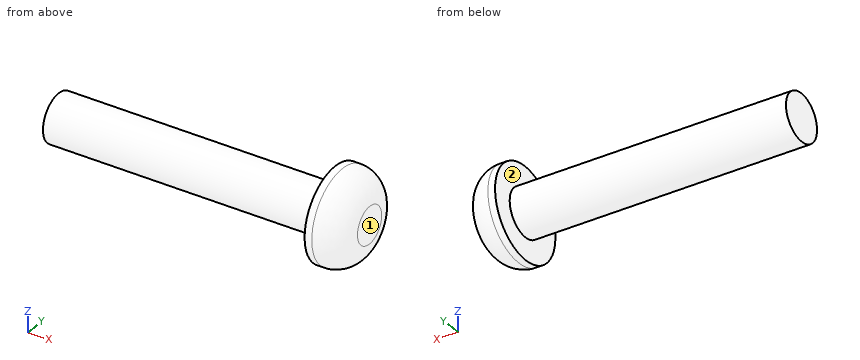
Autodesk Inventor part; units mm, degrees
ref_plane "YZ Plane" through (0, 0, 0) normal (1, 0, 0) x (0, 1, 0)
ref_plane "XZ Plane" through (0, 0, 0) normal (0, 1, 0) x (-1, 0, 0)
ref_plane "XY Plane" through (0, 0, 0) normal (0, 0, 1) x (1, 0, 0)
sketch "Sketch1" plane through (0, 0, 0) normal (1, 0, 0) x (0, 1, 0)
  circle A0 centre (0, 0) radius 1.0922
  dimension "d0" = 2.1844
extrude "Extrusion1" add sketch "Sketch1" along normal blind 12.7
sketch "Sketch2" plane through (12.7, 0, 0) normal (1, 0, 0) x (0, 0, -1)
  circle A0 centre (0, 0) radius 2.1209
  dimension "d3" = 4.2418
extrude "Extrusion2" add sketch "Sketch2" along normal blind 1.6002
fillet "Fillet1" radius 1.27 1 edges at (14.3002, 0, 2.1209)
thread "Thread1"
properties part number "2-56 screw"
Source: CAD feature listing. Evaluate the final solid. Frame: model axes, mm. Face numbers are marked on the shaded views. A direction names the side the tool comes from. Round coordinates to 2 decimals unless told otherwise and drop trailing zeros. Loops run counter-clockwise (first coordinate to the right, second up) from the corner with the lowest first, then second, coordinate; pieces in that order, holes last. Notation, with made-up numbers: M -9.75,-18 L 19.25,-18 A33 ccw 19.25,15 Z; hole C 27,-15.75 d11. An arc over 180 degrees is marked long. Return JSON: item names as keys, results as strings. Group by question number.
1. Section query A-A on x = 9.5. Output: boundary loops of the cut face in (y, z).
2. Pin query (flat end, axial travel): pin 1 (2 mm diameter, centred on x = 2.5, y = -0.5, fed in from -Z); pin 2 (1.3 mm diameter, centred on y = 0, z = 0, fed in from -X); pin 3 (1.5 mm diameter, centred on x = 5.5, z = -1, fed in from +Y). Return the tip coordinate at first contact, or that it passes through.
3. Reachability of the marked faces 1 and 2 from +Z, -Z, +X, -X, +Y, -Y: full face, straight path, thin tool, end or side. Return the list, or none.
4. Material intervals for line 1 along X through (y, z) = (-0.05, -0.9); line 2 along Y through (x, z) = (13, 0.1); line 3 along X through (y, z) = (0.75, 1.2), sorted ascending. Write a range as from..to.
Checks:
{
 "1": {"outline": "C 0,0 d2.18"},
 "2": {"pin 1": "stops at z = -1.09", "pin 2": "stops at x = 0", "pin 3": "stops at y = 1.06"},
 "3": {"face 1": "+Z, -Z, +X, +Y, -Y", "face 2": "-X"},
 "4": {"line 1": "x = 0..14.3", "line 2": "y = -2.12..2.12", "line 3": "x = 12.7..14.17"}
}
